from build123d import *

# Parameters (mm, degrees)
BOSS_EXTRUDE1_DEPTH  = 89.8
SKETCH5_R            = 2.85
BOSS_EXTRUDE2_DEPTH  = 4
SKETCH6_W            = 25
SKETCH6_H            = 11
CUT_EXTRUDE4_DEPTH   = 5
SKETCH8_W            = 19.5
SKETCH8_H            = 4.7
SKETCH8_W_2          = 17.5
SKETCH8_H_2          = 2.7
BOSS_EXTRUDE3_DEPTH  = 15
BOSS_EXTRUDE4_DEPTH  = 19.5
SKETCH13_W           = 17.5
SKETCH13_H           = 2.7
CUT_EXTRUDE5_DEPTH   = 5
SKETCH14_W           = 12.1
SKETCH14_H           = 16.1
SKETCH14_R           = 3.05
BOSS_EXTRUDE7_DEPTH  = 3
CHAMFER1_SIZE        = 3
SKETCH17_R           = 2.1
CUT_EXTRUDE6_DEPTH   = 5
BOSS_EXTRUDE8_DEPTH  = 7
CUT_EXTRUDE7_REACH   = 22.21
SKETCH20_R           = 20.7
FILLET1_R            = 4
SKETCH21_R           = 2.1
CUT_EXTRUDE8_DEPTH   = 5
SKETCH22_W           = 5
SKETCH22_H           = 3
CUT_EXTRUDE9_DEPTH   = 5
BOSS_EXTRUDE9_DEPTH  = 12
FILLET2_R            = 1
FILLET2_OF_MIRROR3_R = 1


with BuildPart() as part:
    # Sketch1 → Boss-Extrude1 (new body)
    with BuildSketch(Plane.XY):
        Polygon((-18, 114.78957189), (0, 114.78957189), (18, 114.78957189), (18, 121.78957189), (16, 121.78957189), (16, 118.78957189), (-16, 118.78957189), (-16, 121.78957189), (-18, 121.78957189), align=None)
    extrude(amount=BOSS_EXTRUDE1_DEPTH)

    # Sketch5 → Boss-Extrude2 (add)
    with BuildSketch(Plane.XY):
        Polygon((-18, 114.78957189), (-18, 131.151236874), (0, 135), (18, 131.151236874), (18, 114.78957189), align=None)
        with Locations((0, 127)):
            Circle(SKETCH5_R, mode=Mode.SUBTRACT)
    boss_extrude2 = extrude(amount=BOSS_EXTRUDE2_DEPTH)

    # Mirror1: Boss-Extrude2 across plane
    add(boss_extrude2.mirror(Plane(origin=(0, 0, 44.9), x_dir=(1, 0, 0), z_dir=(0, 0, -1))))

    # Sketch6 → Cut-Extrude4 (cut, through all)
    with BuildSketch(Plane(origin=(0, 118.78957189, 0), x_dir=(1, 0, 0), z_dir=(0, 1, 0))):
        with Locations((0, -13.5)):
            Rectangle(SKETCH6_W, SKETCH6_H)
    extrude(amount=-CUT_EXTRUDE4_DEPTH, mode=Mode.SUBTRACT)

    # Sketch8 → Boss-Extrude3 (add)
    with BuildSketch(Plane(origin=(0, 118.78957189, 0), x_dir=(1, 0, 0), z_dir=(0, 1, 0))):
        with Locations((0, -74.45)):
            Rectangle(SKETCH8_W, SKETCH8_H)
        with Locations((0, -74.45)):
            Rectangle(SKETCH8_W_2, SKETCH8_H_2, mode=Mode.SUBTRACT)
    extrude(amount=BOSS_EXTRUDE3_DEPTH)

    # Sketch9 → Boss-Extrude4 (add)
    with BuildSketch(Plane.ZY.offset(9.75)):
        Polygon((72.1, 128.78957189), (67.1, 133.78957189), (72.1, 133.78957189), align=None)
    extrude(amount=-BOSS_EXTRUDE4_DEPTH)

    # Sketch13 → Cut-Extrude5 (cut, through all)
    with BuildSketch(Plane(origin=(0, 118.78957189, 0), x_dir=(1, 0, 0), z_dir=(0, 1, 0))):
        with Locations((0, -74.45)):
            Rectangle(SKETCH13_W, SKETCH13_H)
    extrude(amount=-CUT_EXTRUDE5_DEPTH, mode=Mode.SUBTRACT)

    # Sketch14 → Boss-Extrude7 (add)
    with BuildSketch(Plane(origin=(0, 114.78957189, 0), x_dir=(1, 0, 0), z_dir=(0, 1, 0))):
        with Locations((-24.05, -12.05)):
            Rectangle(SKETCH14_W, SKETCH14_H)
        with Locations((-24.05, -12.05)):
            Circle(SKETCH14_R, mode=Mode.SUBTRACT)
    boss_extrude7 = extrude(amount=BOSS_EXTRUDE7_DEPTH)

    # Mirror2: Boss-Extrude7 across plane
    add(boss_extrude7.mirror(Plane(origin=(0, 0, 0), x_dir=(0, 0, 1), z_dir=(1, 0, 0))))

    # Chamfer1
    chamfer1_edges = [part.edges().sort_by_distance(p)[0] for p in [
        (-18, 116.28957189, 20.1),
        (-18, 116.28957189, 4),
        (18, 116.28957189, 4),
        (18, 116.28957189, 20.1),
    ]]
    chamfer(chamfer1_edges, length=CHAMFER1_SIZE)

    # Sketch17 → Cut-Extrude6 (cut, through all)
    with BuildSketch(Plane(origin=(0, 118.78957189, 0), x_dir=(1, 0, 0), z_dir=(0, 1, 0))):
        with Locations((0, -81.15)):
            Circle(SKETCH17_R)
    extrude(amount=-CUT_EXTRUDE6_DEPTH, mode=Mode.SUBTRACT)

    # Sketch19 → Boss-Extrude8 (add)
    with BuildSketch(Plane.XZ.offset(-114.78957189)):
        with BuildLine():
            Line((18, 67.25374689), (18, 55.122035022))
            ThreePointArc((18, 55.122035022), (20.7, 44.9), (18, 34.677964978))
            Line((18, 34.677964978), (18, 22.54625311))
            ThreePointArc((18, 22.54625311), (28.7, 44.9), (18, 67.25374689))
        make_face()
        with BuildLine():
            Line((-16, 68.726246032), (-16, 58.033544838))
            ThreePointArc((-16, 58.033544838), (-20.624518846, 46.666132031), (-18, 34.677964978))
            Line((-18, 34.677964978), (-18, 22.54625311))
            ThreePointArc((-18, 22.54625311), (-28.673122198, 46.141798467), (-16, 68.726246032))
        make_face()
    extrude(amount=-BOSS_EXTRUDE8_DEPTH)

    # Sketch20 → Cut-Extrude7 (cut, up to next)
    with BuildSketch(Plane.XZ.offset(-114.78957189), mode=Mode.PRIVATE) as cut_extrude7_sk1:
        with Locations((0, 44.9)):
            Circle(SKETCH20_R)
    cut_extrude7_tool1 = extrude(cut_extrude7_sk1.sketch, amount=-CUT_EXTRUDE7_REACH, mode=Mode.PRIVATE) & part.part
    add(cut_extrude7_tool1.solids().sort_by_distance((0, 114.789572, 44.9))[0], mode=Mode.SUBTRACT)

    # Fillet1
    fillet1_edges = [part.edges().sort_by_distance(p)[0] for p in [
        (-30.1, 116.28957189, 4),
        (-30.1, 116.28957189, 20.1),
        (30.1, 116.28957189, 20.1),
        (30.1, 116.28957189, 4),
    ]]
    fillet(fillet1_edges, radius=FILLET1_R)

    # Sketch21 → Cut-Extrude8 (cut, through all)
    with BuildSketch(Plane(origin=(0, 118.78957189, 0), x_dir=(1, 0, 0), z_dir=(0, 1, 0))):
        with Locations((-10.26962376, -66.923279225)):
            Circle(SKETCH21_R)
        with Locations((10.26962376, -66.923279225)):
            Circle(SKETCH21_R)
    extrude(amount=-CUT_EXTRUDE8_DEPTH, mode=Mode.SUBTRACT)

    # Sketch22 → Cut-Extrude9 (cut, through all)
    with BuildSketch(Plane(origin=(0, 118.78957189, 0), x_dir=(1, 0, 0), z_dir=(0, 1, 0))):
        with Locations((0, -66.948479262)):
            Rectangle(SKETCH22_W, SKETCH22_H)
        with Locations((0, -22.851520738)):
            Rectangle(SKETCH22_W, SKETCH22_H)
    extrude(amount=-CUT_EXTRUDE9_DEPTH, mode=Mode.SUBTRACT)

    # Sketch23 → Boss-Extrude9 (add)
    with BuildSketch(Plane(origin=(0, 121.78957189, 0), x_dir=(1, 0, 0), z_dir=(0, 1, 0))):
        Polygon((-18.7, -26.9), (-16, -26.9), (-16, -28.4), (-17.2, -28.4), (-17.2, -33.382621826), (-18.7, -33.382621826), align=None)
    boss_extrude9 = extrude(amount=BOSS_EXTRUDE9_DEPTH)

    # Fillet2
    fillet2_edges = [part.edges().sort_by_distance(p)[0] for p in [
        (-16, 127.78957189, 26.9),
        (-18.7, 127.78957189, 33.382621826),
        (-18.7, 127.78957189, 26.9),
    ]]
    fillet(fillet2_edges, radius=FILLET2_R)

    # Mirror3: Boss-Extrude9 across plane
    add(boss_extrude9.mirror(Plane(origin=(0, 0, 0), x_dir=(0, 0, 1), z_dir=(1, 0, 0))))

    # Fillet2 of Mirror3
    fillet2_of_mirror3_edges = [part.edges().sort_by_distance(p)[0] for p in [
        (16, 127.78957189, 26.9),
        (18.7, 127.78957189, 33.382621826),
        (18.7, 127.78957189, 26.9),
    ]]
    fillet(fillet2_of_mirror3_edges, radius=FILLET2_OF_MIRROR3_R)


solid = part.part
Design review of the part built by this model. Coordinates are the model's own, in mm. A direction names the side the tool comes from. Coordinates: 2 decimals unless noted, no trailing zeros. Write each loop counter-clockwise with the first axis right and the second up, starting at its lowest first coordinate (ties: lowest second). Pieces come first, ordered by that corner, then holes. Notation, with made-up numbers: (65.5, 77.25) -> (112.5, 77.25) arc R24 cw to (112.5, 100.25) -> close; hole circle Ø4 at (79, 54.25). An arc over 180 degrees is marked (long way). Write each question's results on one line, items separated by ' | '. Start each with the question number.
(1) Take a section at D-D on x = -24.05. Write out the cut boundary in (y, z).
(2) Take a section at B-B on z = 12.05. Write out the cut boundary in (x, y).
(3) The part is to be moulded in two halves that separate along X. For faces 1 (the face through (-21, 117.79, 14)), 2 (the face through (28.698, 118.241, 44.541)), 3 (the face through (8.75, 124, 74)), 4 (the face through (-18, 121, 9)), say which applies: pulls with the +X half, pulls with the -X half, needs draft (parallel to the pull), parting line crosses it, or undercut.
(4) For line 1 along Z through (x, y) = (1, 121.5); line 2 along Z through (x, y) = (0, 117.75); line 3 along X through (y, z) = (116.45, 12.05), list the stretches that pass through material, from the lowest coordinate up. Write a range as from..to.
(5) Take a section at C-C on z = 81.15. Write out the cut boundary in (x, y).
(6) Take a section at A-A on y = 120.25. Write out the cut boundary in (x, z), and give its area (3 significant figures).
(7) Clearance check with flat-ended pins moving along their axes: P1, Ø8, axis at x = 17.5, z = 61, coming from the +Y side; P2, Ø2, axis at y = 125.5, z = 29, coming from the +X side; P3, Ø12, axis at x = -24, z = 33.5, coming from the +Y side. State where each tip first meets the part, or that it passes through.
(8) Tool access review of faces 5 (the face through (9.75, 128, 74)), 6 (the face through (-24, 116, 20.1)), 7 (the face through (-9.126, 133.049, 1.972)), 8 (the face through (0, 118.79, 78)): name each direction out of +Z, -Z, +X, -X, +Y, -Y from which nothing blocks a thin tool from reaching the whole face with its end or side.
Results found:
1) outline: (114.79, 4) -> (117.79, 4) -> (117.79, 9) -> (114.79, 9) -> close; (114.79, 15.1) -> (117.79, 15.1) -> (117.79, 20.1) -> (114.79, 20.1) -> close; (114.79, 29.24) -> (121.79, 29.24) -> (121.79, 60.56) -> (114.79, 60.56) -> close
2) outline: (-30.1, 114.79) -> (-27.1, 114.79) -> (-27.1, 117.79) -> (-30.1, 117.79) -> close; (-21, 114.79) -> (-12.5, 114.79) -> (-12.5, 118.79) -> (-16, 118.79) -> (-16, 121.79) -> (-18, 121.79) -> (-18, 117.79) -> (-21, 117.79) -> close; (12.5, 114.79) -> (21, 114.79) -> (21, 117.79) -> (18, 117.79) -> (18, 121.79) -> (16, 121.79) -> (16, 118.79) -> (12.5, 118.79) -> close; (27.1, 114.79) -> (30.1, 114.79) -> (30.1, 117.79) -> (27.1, 117.79) -> close
3) face 1: needs draft | face 2: pulls with the +X half | face 3: undercut | face 4: pulls with the -X half
4) line 1: z = 0..4, 72.1..73.1, 75.8..76.8, 85.8..89.8 | line 2: z = 0..8, 19..21.35, 68.45..73.1, 75.8..79.05, 83.25..89.8 | line 3: x = -30.1..-27.1, -21..-12.5, 12.5..21, 27.1..30.1
5) outline: (-18, 114.79) -> (-2.1, 114.79) -> (-2.1, 118.79) -> (-16, 118.79) -> (-16, 121.79) -> (-18, 121.79) -> close; (2.1, 114.79) -> (18, 114.79) -> (18, 121.79) -> (16, 121.79) -> (16, 118.79) -> (2.1, 118.79) -> close
6) outline: (-18, 0) -> (18, 0) -> (18, 22.55) arc R28.7 ccw to (18, 67.25) -> (18, 89.8) -> (-18, 89.8) -> (-18, 67.25) arc R28.7 ccw to (-18, 22.55) -> close; (-9.75, 72.1) -> (9.75, 72.1) -> (9.75, 76.8) -> (-9.75, 76.8) -> close; hole (-16, 4) -> (16, 4) -> (16, 31.77) arc R20.7 ccw to (16, 58.03) -> (16, 85.8) -> (-16, 85.8) -> (-16, 58.03) arc R20.7 ccw to (-16, 31.77) -> close; hole (-8.75, 73.1) -> (8.75, 73.1) -> (8.75, 75.8) -> (-8.75, 75.8) -> close | area: 1,160 mm2
7) P1: stops at y = 121.79 | P2: stops at x = 18.7 | P3: stops at y = 133.79
8) face 5: +Y | face 6: -X, +Y, -Y | face 7: -Z, -X, +Y | face 8: none
